The model under review builds one solid part; all positions refer to its coordinate system, in mm. Face numbers are marked on the shaded views. Coordinates: 2 decimals unless noted, no trailing zeros. Write each loop counter-clockwise with the first axis right and the second up, starting at its lowest first coordinate (ties: lowest second). Pieces come first, ordered by that corner, then holes.
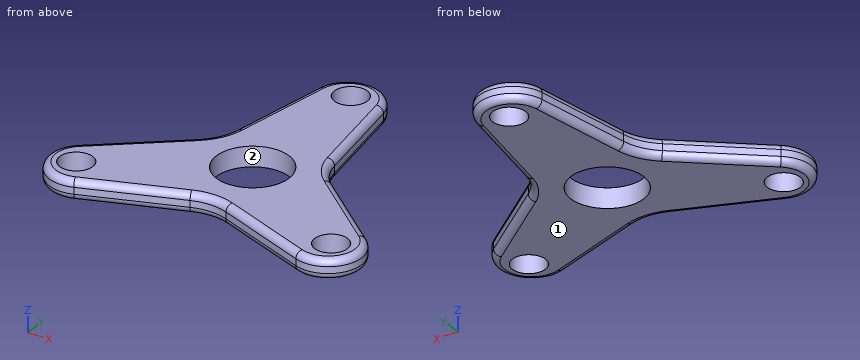
```python
from build123d import *

# Parameters (mm, degrees)
F0_R     = 5
F0_R_2   = 11
F1_DEPTH = 6
F2_R     = 2


with BuildPart() as f1:
    # F0 (on Top) → F1 (new body)
    with BuildSketch(Plane.XY):
        with BuildLine():
            ThreePointArc((10, 44.979472), (0, 53.449789), (-10, 44.979472))
            Line((-10, 44.979472), (-15, 15))
            ThreePointArc((-15, 15), (-16.884039, 9.748004), (-20.490381, 5.490381))
            Line((-20.490381, 5.490381), (-43.953365, -13.829482))
            ThreePointArc((-43.953365, -13.829482), (-46.288875, -26.724895), (-33.953365, -31.14999))
            Line((-33.953365, -31.14999), (-5.490381, -20.490381))
            ThreePointArc((-5.490381, -20.490381), (0, -19.496009), (5.490381, -20.490381))
            Line((5.490381, -20.490381), (33.953365, -31.14999))
            ThreePointArc((33.953365, -31.14999), (46.288875, -26.724895), (43.953365, -13.829482))
            Line((43.953365, -13.829482), (20.490381, 5.490381))
            ThreePointArc((20.490381, 5.490381), (16.884039, 9.748004), (15, 15))
            Line((15, 15), (10, 44.979472))
        make_face()
        with Locations((-38.971143, -22.5)):
            Circle(F0_R, mode=Mode.SUBTRACT)
        with Locations((38.971143, -22.5)):
            Circle(F0_R, mode=Mode.SUBTRACT)
        Circle(F0_R_2, mode=Mode.SUBTRACT)
        with Locations((0, 45)):
            Circle(F0_R, mode=Mode.SUBTRACT)
    extrude(amount=F1_DEPTH)

    # F2
    f2_edges = [f1.edges().sort_by_distance(p)[0] for p in [
        (-12.5, 29.989736, 6),
        (-12.5, 29.989736, 0),
    ]]
    fillet(f2_edges, radius=F2_R)


solid = f1.part
```
Item 1: For pin 1 (2 mm diameter, centred on x = -30, z = 0.5, fed in from -Y); pin 2 (1 mm diameter, centred on x = -1.5, z = 5, fed in from -Y), all flat-tipped, find the tip position at first contact; note any pin that passes through.
Solved:
pin 1: stops at y = -29.76
pin 2: stops at y = -19.51
Item 2: To check wall thickness, follow line 1 along X through (y, z) = (-18.5, 2.5); line 2 along Y through (x, z) = (41.5, 4.5); line 3 along X through (y, z) = (7, 3.25). State the ranges of each line that lie inside material, in increasing order.
Solved:
line 1: x = -47.14 to -41.97, -35.97 to 35.97, 41.97 to 47.14
line 2: y = -30.91 to -26.81, -18.19 to -11.89
line 3: x = -18.9 to -8.49, 8.49 to 18.9
Item 3: Take a section at B-B, the plane z = 3. Write out the cut boundary in (x, y), plus the area to 3 significant figures.
Solved:
outline: (-43.95, -13.83) arc R10.14 ccw to (-33.95, -31.15) - (-5.49, -20.49) arc R15.65 cw to (5.49, -20.49) - (33.95, -31.15) arc R10.14 ccw to (43.95, -13.83) - (20.49, 5.49) arc R15.65 cw to (15, 15) - (10, 44.98) arc R10.14 ccw to (-10, 44.98) - (-15, 15) arc R15.65 cw to (-20.49, 5.49) - close; hole circle Ø10 at (-38.97, -22.5); hole circle Ø22 at (0, 0); hole circle Ø10 at (0, 45); hole circle Ø10 at (38.97, -22.5)
area: 3,010 mm2
Item 4: Take a section at C-C, the plane y = -22.5. Count the separate pieces of the cut face and the enclosed holes in it, plus the area to 3 significant figures.
Solved:
separate pieces: 4
enclosed holes: 0
area: 308 mm2
Item 5: Take a section at A-A, the plane x = 0. Write out the cut boundary in (y, z), plus the area to 3 significant figures.
Solved:
outline: (-19.5, 2) arc R2 ccw to (-17.5, 0) - (-11, 0) - (-11, 6) - (-17.5, 6) arc R2 ccw to (-19.5, 4) - close; (11, 0) - (40, 0) - (40, 6) - (11, 6) - close; (50, 0) - (51.45, 0) arc R2 ccw to (53.45, 2) - (53.45, 4) arc R2 ccw to (51.45, 6) - (50, 6) - close
area: 242 mm2
Item 6: Mouldability with a two-part tool opening along Y and no side actions: class the marked faces 1 and 2 as pulls with the +Y half, pulls with the -Y half, needs draft (parallel to the pull), parting line crosses it, or undercut.
Solved:
face 1: needs draft
face 2: undercut
